Design review of the part built by this model. Coordinates are the model's own, in mm. Face numbers are marked on the shaded views. A direction names the side the tool comes from. Give positions to 0.01 mm unless a question says otherwise; leave off trailing zeros. Order: outer loops, then holes, each group sorted by start corner. A loop starts at its lowest first (then second) coordinate and runs counter-clockwise, first axis right, second up. Notation, with made-up numbers: (61.5, 5) -> (75.5, 5) arc R26 ccw to (75.5, 39) -> close; hole circle Ø10 at (19.25, 84). An arc over 180 degrees is marked (long way). One line per item, written item: value. Start each with the question number.
1) Tool access review of the marked faces 1 and 2: name each direction out of +Z, -Z, +X, -X, +Y, -Y from which nothing blocks a thin tool from reaching the whole face with its end or side.
2) The part is to be moulded in two halves that separate along Z. For the marked faces 3, 4, 5 and 6, say which applies: released by +Z, released by -Z, zero draft, split by the parting line, or undercut.
3) Consider section A-A (z = 11). State the section outline as (x, y) points.
4) Wall thickness on line 1 along X through (y, z) = (-85.5, -1.5); line 2 along Y through (x, z) = (-18.25, 0): over which ranges is each line inside the solid? List them lowest first. Write a range as from..to.
5) Consider section B-B (x = -13). State the section outline as (y, z) points.
6) Consider section C-C (y = -163). State the section outline as (x, z) points.
from build123d import *

# Parameters (mm, degrees)
F2_W            = 40
F2_H            = 40
F3_DEPTH        = 240
F4_R            = 3
F5_T            = -2
F7_DEPTH        = 40.001
F9_DEPTH        = 40.001
F11_D           = 3.5
F11_CSINK_D     = 6
F11_CSINK_ANGLE = 90


with BuildPart() as f3:
    # F2 (on Front) → F3 (new body, symmetric)
    with BuildSketch(Plane.XZ):
        Rectangle(F2_W, F2_H)
    extrude(amount=F3_DEPTH, both=True)

    # F4
    f4_edges = [f3.edges().sort_by_distance(p)[0] for p in [
        (20, 0, 20),
        (-20, 0, 20),
        (20, 0, -20),
        (-20, 0, -20),
    ]]
    fillet(f4_edges, radius=F4_R)

    # F5
    f5_openings = [f3.faces().sort_by_distance(p)[0] for p in [
        (0, -240, 0),
        (0, 240, 0),
    ]]
    offset(amount=F5_T, openings=f5_openings)

    # F6 (on face) → F7 (cut, through all)
    with BuildSketch(Plane(origin=(-20, 0, 0), x_dir=(0, -1, 0), z_dir=(-1, 0, 0))):
        Polygon((-240, 20), (-240, -20), (-200, -20), align=None)
    extrude(amount=-F7_DEPTH, mode=Mode.SUBTRACT)

    # F8 (on face) → F9 (cut, through all)
    with BuildSketch(Plane.XY.offset(20)):
        Polygon((-20, -200), (-20, -240), (20, -240), align=None)
    extrude(amount=-F9_DEPTH, mode=Mode.SUBTRACT)

    # F11 (through all)
    with Locations(Plane(origin=(-20, 0, 0), x_dir=(0, -1, 0), z_dir=(-1, 0, 0))):
        with Locations((-180, 0), (-60, 0), (60, 0), (180, 0)):
            CounterSinkHole(F11_D / 2, F11_CSINK_D / 2, counter_sink_angle=F11_CSINK_ANGLE)


solid = f3.part
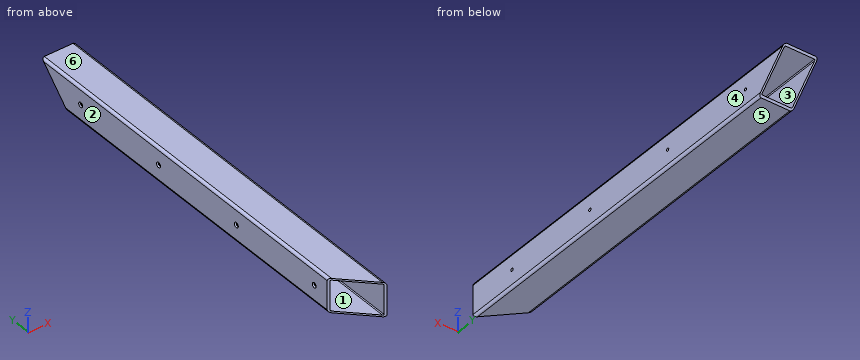
Checked values:
1. face 1: +Y, -Y
1. face 2: +Z, -Z, -X, +Y, -Y
2. face 3: undercut
2. face 4: zero draft
2. face 5: released by -Z
2. face 6: released by +Z
3. outline: (-20, -200) -> (-18, -202) -> (-18, 231) -> (-20, 231) -> close; (18, -238) -> (20, -240) -> (20, 231) -> (18, 231) -> close
4. line 1: x = -20..-18, 18..20
4. line 2: y = -201.75..-181.75, -178.25..-61.75, -58.25..58.25, 61.75..178.25, 181.75..220
5. outline: (-207, -20) -> (200, -20) -> (202, -18) -> (-207, -18) -> close; (-207, 18) -> (238, 18) -> (240, 20) -> (-207, 20) -> close
6. outline: (-20, -17) arc R3 ccw to (-17, -20) -> (17, -20) arc R3 ccw to (20, -17) -> (20, 17) arc R3 ccw to (17, 20) -> (-17, 20) arc R3 ccw to (-20, 17) -> close; hole (-18, -17) arc R1 ccw to (-17, -18) -> (17, -18) arc R1 ccw to (18, -17) -> (18, 17) arc R1 ccw to (17, 18) -> (-17, 18) arc R1 ccw to (-18, 17) -> close
